Autodesk Inventor part; units mm, degrees
ref_plane "YZ Plane" through (0, 0, 0) normal (1, 0, 0) x (0, 1, 0)
ref_plane "XZ Plane" through (0, 0, 0) normal (0, 1, 0) x (-1, 0, 0)
ref_plane "XY Plane" through (0, 0, 0) normal (0, 0, 1) x (1, 0, 0)
sketch "Sketch1" plane through (0, 0, 0) normal (0, 0, 1) x (1, 0, 0)
  line L0 (0, 0) -> (50.8, 0)
  line L1 (50.8, 0) -> (50.8, 76.2)
  line L2 (50.8, 76.2) -> (0, 76.2)
  line L3 (0, 76.2) -> (0, 0)
  line L4 (3.175, 73.025) -> (47.625, 73.025)
  line L5 (47.625, 73.025) -> (47.625, 3.175)
  line L6 (47.625, 3.175) -> (3.175, 3.175)
  line L7 (3.175, 3.175) -> (3.175, 73.025)
  dimension "d13" = 3.175
  dimension "d14" = 50.8
  dimension "d15" = 76.2
  dimension "d16" = 3.175
  dimension "d17" = 3.175
  dimension "d18" = 3.175
extrude "Extrusion1" add sketch "Sketch1" along normal blind 1498.6
properties part number "GE-12019-05" material "Aluminum-6061"
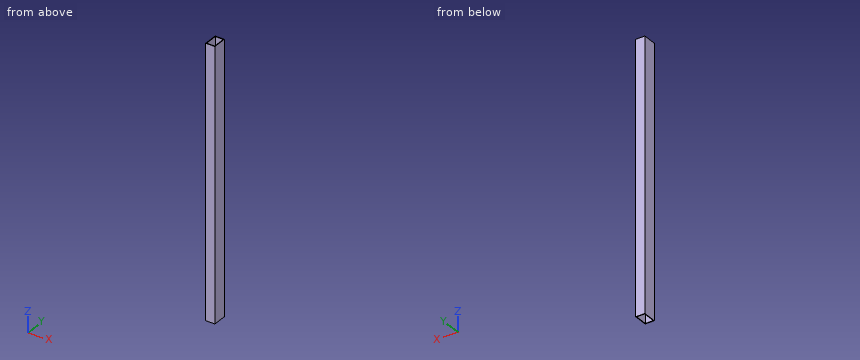
Read the model definition and answer for the solid it produces. Units are mm, in the model's axes. Coordinates: 2 decimals unless noted, no trailing zeros. Order: outer loops, then holes, each group sorted by start corner. A loop starts at its lowest first (then second) coordinate and runs counter-clockwise, first axis right, second up. Notation, with made-up numbers: (-29.75, 2) - (-21.75, 2) arc R19 ccw to (-21.75, 27) - close; hole circle Ø7 at (78, 36). An arc over 180 degrees is marked (long way). Answer as a JSON object with one key per item and string values. Group by question number.
Item 1: Consider probe 1 along Y at (x, z) = (47.5, 1142.5) (3 decimals); probe 2 along X at (y, z) = (71, 768.5) (3 decimals). Determine where each line is inside the solid, lowest interval first. Write a range as from..to.
Item 2: Section C-C (z = 754) is taken. Give the vertices of the cut face in (x, y) (3 decimals), plus the area to 3 significant figures.
Item 3: Section A-A (y = 21.5) is taken. Give the vertices of the cut face in (x, z) (3 decimals), plus the area to 3 significant figures.
Item 4: Section B-B (x = 35.5) is taken. Give the vertices of the cut face in (y, z) (3 decimals), plus the area to 3 significant figures.
Results are:
{
 "1": {"probe 1": "y = 0..3.175, 73.025..76.2", "probe 2": "x = 0..3.175, 47.625..50.8"},
 "2": {"outline": "(0, 0) - (50.8, 0) - (50.8, 76.2) - (0, 76.2) - close; hole (3.175, 3.175) - (47.625, 3.175) - (47.625, 73.025) - (3.175, 73.025) - close", "area": "766 mm^2"},
 "3": {"outline": "(0, 0) - (3.175, 0) - (3.175, 1498.6) - (0, 1498.6) - close; (47.625, 0) - (50.8, 0) - (50.8, 1498.6) - (47.625, 1498.6) - close", "area": "9,520 mm^2"},
 "4": {"outline": "(0, 0) - (3.175, 0) - (3.175, 1498.6) - (0, 1498.6) - close; (73.025, 0) - (76.2, 0) - (76.2, 1498.6) - (73.025, 1498.6) - close", "area": "9,520 mm^2"}
}
